```python
from build123d import *

# Parameters (mm, degrees)
SKETCH1_R           = 35.304197416
BOSS_EXTRUDE1_DEPTH = 10
SKETCH2_R           = 18.229259508
BOSS_EXTRUDE2_DEPTH = 100
CHAMFER1_SIZE       = 10
CHAMFER1_SIZE2      = 16.00334529


with BuildPart() as part:
    # Sketch1 → Boss-Extrude1 (new body)
    with BuildSketch(Plane.XY):
        Circle(SKETCH1_R)
    extrude(amount=BOSS_EXTRUDE1_DEPTH)

    # Sketch2 → Boss-Extrude2 (add)
    with BuildSketch(Plane.XY.offset(10)):
        with Locations(Location((0, 0, 0), (0, 0, 180))):
            Circle(SKETCH2_R)
    extrude(amount=BOSS_EXTRUDE2_DEPTH)

    # Chamfer1
    chamfer1_edges = [part.edges().sort_by_distance(p)[0] for p in [
        (18.229259508, 0, 110),
    ]]
    chamfer1_side = [part.faces().sort_by_distance(p)[0] for p in [
        (18.229259508, 0, 60),
    ]]
    chamfer(chamfer1_edges, length=CHAMFER1_SIZE, length2=CHAMFER1_SIZE2, reference=chamfer1_side[0])


solid = part.part
```
The listing builds one solid part. Answer for the finished solid, in the listing's coordinates (mm). A direction names the side the tool comes from. Round coordinates to 2 decimals unless told otherwise and drop trailing zeros. Loops run counter-clockwise (first coordinate to the right, second up) from the corner with the lowest first, then second, coordinate; pieces in that order, holes last.
Q1. Section C-C, the plane z = 28 is taken. Determine the outline of the cut face in (x, y).
Q2. Section D-D, the plane x = -26.5 is taken. Determine the outline of the cut face in (y, z).
Q3. Given pin 1 Ø5 at (y, z) = (18.5, 52) entering from +X; pin 2 Ø3 at (y, z) = (-15, 15) entering from -X; pin 3 Ø10 at (y, z) = (-9, 23) entering from +X (3 decimals); pin 4 Ø10 at (y, z) = (25.5, 62.5) entering from +X (3 decimals), each flat-ended and moving along its own axis, determine where each tip first touches the part or whether it passes through.
Q4. Section A-A, the plane x = 0 is taken. Determine the outline of the cut face in (y, z), then the cut area to 3 significant figures.
Q5. Find the intervals of material crossed by line 1 (Z direction, x = 14, y = -16); line 2 (X direction, y = -0.5, z = 21.5); line 3 (Y direction, x = 1, z = 38.5), in increasing order.
Q6. Which of the six approach directions +Z, -Z, +X, -X, +Y, -Y give full straight-line access (tool end or side, diameter ignored) to faces 1 (the face through (0, 0, 110)), 2 (the face through (2.373, -18.074, 54.37))?
Completed:
1. outline: circle Ø36.46 at (0, 0)
2. outline: (-23.33, 0) - (23.33, 0) - (23.33, 10) - (-23.33, 10) - close
3. pin 1: stops at x = 8.74
3. pin 2: stops at x = -12.25
3. pin 3: stops at x = 17.785
3. pin 4: passes through
4. outline: (-35.3, 0) - (35.3, 0) - (35.3, 10) - (18.23, 10) - (18.23, 100) - (2.23, 110) - (-2.23, 110) - (-18.23, 100) - (-18.23, 10) - (-35.3, 10) - close
4. area: 4,190 mm2
5. line 1: z = 0 to 10
5. line 2: x = -18.22 to 18.22
5. line 3: y = -18.2 to 18.2
6. face 1: +Z, +X, -X, +Y, -Y
6. face 2: +Z
